Source: CAD feature listing. Evaluate the final solid. Frame: model axes, mm. Give positions to 0.01 mm unless a question says otherwise; leave off trailing zeros. Answer as a JSON object with one key per item and string values. Group by question number.
1. Pin query (flat end, axial travel): P1, Ø5, axis at x = -78.5, z = -41.5, coming from the -Y side. Return the tip coordinate at first contact, or that it passes through.
2. Pull-direction query (Z, two-part tool) for faces 1 (the cylindrical face through (53.393, 71.479, 44.233)), 2 (the flat face through (-13, 73, -1)), 3 (the cylindrical face through (56.797, 71.479, 44.359)), 4 (the cylindrical face through (56.859, 71.479, -44.297)); classes: +Z half, -Z half, draft (parallel to the pull), parting line (faces both ways), or undercut.
3. Material intervals for L1, parallel to X at y = 72.05, z = 41.5; L2, parallel to Z at x = -78.5, y = 72.05, sorted ascending. Write a range as [from, to].
from build123d import *

# Parameters (mm, degrees)
SKETCH1_W                 = 134.5
SKETCH1_H                 = 85
BOSS_EXTRUDE1_DEPTH       = 3
SKETCH2_W                 = 140.5
SKETCH2_H                 = 91
SKETCH2_W_2               = 134.5
SKETCH2_H_2               = 85
BOSS_EXTRUDE2_DEPTH       = 70
BOSS_EXTRUDE3_START       = 5
SKETCH3_W                 = 100
SKETCH3_H                 = 80
BOSS_EXTRUDE3_DEPTH       = 5
SKETCH5_W                 = 3
SKETCH5_H                 = 66
BOSS_EXTRUDE5_DEPTH       = 30
SKETCH6_R                 = 3
SKETCH6_R_2               = 1
BOSS_EXTRUDE6_DEPTH       = 10
SKETCH7_W                 = 100
SKETCH7_H                 = 80
CUT_EXTRUDE2_DEPTH        = 10
SKETCH6_2_R               = 3
SKETCH6_2_R_2             = 1
BOSS_EXTRUDE7_DEPTH       = 8
MIRROR4_COPY_1_SKETCH_R   = 3
MIRROR4_COPY_1_SKETCH_R_2 = 1
MIRROR4_COPY_1_DEPTH      = 8
SKETCH9_R                 = 26.15
SKETCH9_W                 = 29.3
SKETCH9_H                 = 26.2
SKETCH9_R_2               = 1
SKETCH9_R_3               = 3.4
SKETCH9_R_4               = 7.9
CUT_EXTRUDE3_DEPTH        = 3
SKETCH10_R                = 2.95
SKETCH10_R_2              = 5.9
CUT_EXTRUDE4_DEPTH        = 3
BOSS_EXTRUDE8_DEPTH       = 7
FILLET1_R                 = 4
CUT_EXTRUDE6_DEPTH        = 5
SKETCH14_R                = 2.8
BOSS_EXTRUDE9_DEPTH       = 3


with BuildPart() as part:
    # Sketch1 → Boss-Extrude1 (new body)
    with BuildSketch(Plane(origin=(0, 0, 0), x_dir=(1, 0, 0), z_dir=(0, 1, 0))):
        with Locations((-12.25, 0)):
            Rectangle(SKETCH1_W, SKETCH1_H)
    extrude(amount=BOSS_EXTRUDE1_DEPTH)

    # Sketch2 → Boss-Extrude2 (add)
    with BuildSketch(Plane(origin=(0, 0, 0), x_dir=(1, 0, 0), z_dir=(0, 1, 0))):
        with Locations((-12.25, 0)):
            Rectangle(SKETCH2_W, SKETCH2_H)
        with Locations((-12.25, 0)):
            Rectangle(SKETCH2_W_2, SKETCH2_H_2, mode=Mode.SUBTRACT)
    extrude(amount=BOSS_EXTRUDE2_DEPTH)

    # Sketch5 → Boss-Extrude5 (add)
    with BuildSketch(Plane(origin=(0, 3, 0), x_dir=(1, 0, 0), z_dir=(0, 1, 0))):
        Polygon((-58, -26.5), (-58, -23.5), (-61, -23.5), (-79.5, -23.5), (-79.5, -26.5), align=None)
        with Locations((-59.5, 9.5)):
            Rectangle(SKETCH5_W, SKETCH5_H)
    extrude(amount=BOSS_EXTRUDE5_DEPTH)



with BuildPart() as body_2:
    # Sketch3 → Boss-Extrude3 (new body)
    with BuildSketch(Plane(origin=(0, 3, 0), x_dir=(1, 0, 0), z_dir=(0, 1, 0)).offset(BOSS_EXTRUDE3_START)):
        Rectangle(SKETCH3_W, SKETCH3_H)
    extrude(amount=BOSS_EXTRUDE3_DEPTH)


with BuildPart() as part_1:
    add(part.part)

    add(body_2.part)  # Boss-Extrude6 merges body 2
    # Sketch6 → Boss-Extrude6 (add)
    with BuildSketch(Plane(origin=(0, 3, 0), x_dir=(1, 0, 0), z_dir=(0, 1, 0))):
        with Locations((-45, -35)):
            Circle(SKETCH6_R)
        with Locations((-45, -35)):
            Circle(SKETCH6_R_2, mode=Mode.SUBTRACT)
    extrude(amount=BOSS_EXTRUDE6_DEPTH)

    # Sketch7 → Cut-Extrude2 (cut)
    with BuildSketch(Plane(origin=(0, 13, 0), x_dir=(1, 0, 0), z_dir=(0, 1, 0))):
        Rectangle(SKETCH7_W, SKETCH7_H)
    extrude(amount=-CUT_EXTRUDE2_DEPTH, mode=Mode.SUBTRACT)

    # Sketch6<2> → Boss-Extrude7 (add)
    with BuildSketch(Plane(origin=(0, 3, 0), x_dir=(1, 0, 0), z_dir=(0, 1, 0))):
        with Locations((-45, -35)):
            Circle(SKETCH6_2_R)
        with Locations((-45, -35)):
            Circle(SKETCH6_2_R_2, mode=Mode.SUBTRACT)
    boss_extrude7 = extrude(amount=BOSS_EXTRUDE7_DEPTH)

    # Mirror3: Boss-Extrude7 across plane
    add(boss_extrude7.mirror(Plane.XY))

    # Mirror4: Boss-Extrude7 across plane
    add(boss_extrude7.mirror(Plane(origin=(0, 0, 0), x_dir=(0, 0, 1), z_dir=(1, 0, 0))))

    # Mirror4 copy 1 sketch → Mirror4 copy 1 (add)
    with BuildSketch(Plane(origin=(0, 3, 0), x_dir=(-1, 0, 0), z_dir=(0, 1, 0))):
        with Locations((-45, -35)):
            Circle(MIRROR4_COPY_1_SKETCH_R)
        with Locations((-45, -35)):
            Circle(MIRROR4_COPY_1_SKETCH_R_2, mode=Mode.SUBTRACT)
    extrude(amount=MIRROR4_COPY_1_DEPTH)

    # Sketch9 → Cut-Extrude3 (cut)
    with BuildSketch(Plane.XY.offset(45.5)):
        with Locations((23, 40.85)):
            Circle(SKETCH9_R)
        with Locations((-47.5, 50)):
            Rectangle(SKETCH9_W, SKETCH9_H)
        with Locations((1.786796564, 62.063203436)):
            Circle(SKETCH9_R_2)
        with Locations((44.213203436, 62.063203436)):
            Circle(SKETCH9_R_2)
        with Locations((44.213203436, 19.636796564)):
            Circle(SKETCH9_R_2)
        with Locations((1.786796564, 19.636796564)):
            Circle(SKETCH9_R_2)
        with Locations((-58.75, 21.9)):
            Circle(SKETCH9_R_3)
        with Locations((-40.75, 21.9)):
            Circle(SKETCH9_R_4)
    extrude(amount=-CUT_EXTRUDE3_DEPTH, mode=Mode.SUBTRACT)

    # Sketch10 → Cut-Extrude4 (cut)
    with BuildSketch(Plane(origin=(58, 0, 0), x_dir=(0, 0, -1), z_dir=(1, 0, 0))):
        with Locations((15.5, 55)):
            Circle(SKETCH10_R)
        with Locations((30.5, 55)):
            Circle(SKETCH10_R_2)
    extrude(amount=-CUT_EXTRUDE4_DEPTH, mode=Mode.SUBTRACT)

    # Sketch11 → Boss-Extrude8 (add)
    with BuildSketch(Plane(origin=(0, 70, 0), x_dir=(1, 0, 0), z_dir=(0, 1, 0))):
        Polygon((-74.5, 42.5), (-79.5, 42.5), (-79.5, 37.5), align=None)
        Polygon((55, 37.5), (55, 42.5), (50, 42.5), align=None)
        Polygon((50, -42.5), (55, -42.5), (55, -37.5), align=None)
        Polygon((-79.5, -37.5), (-79.5, -42.5), (-74.5, -42.5), align=None)
    extrude(amount=-BOSS_EXTRUDE8_DEPTH)

    # Fillet1
    fillet1_edges = [part_1.edges().sort_by_distance(p)[0] for p in [
        (58, 35, 45.5),
        (58, 35, -45.5),
        (-82.5, 35, -45.5),
        (-82.5, 35, 45.5),
    ]]
    fillet(fillet1_edges, radius=FILLET1_R)

    # Sketch13 → Cut-Extrude6 (cut)
    with BuildSketch(Plane(origin=(0, 70, 0), x_dir=(1, 0, 0), z_dir=(0, 1, 0))):
        with BuildLine():
            ThreePointArc((55.371320344, 42.871320344), (53.957106781, 42.871320344), (53.957106781, 41.457106781))
            Line((53.957106781, 41.457106781), (55.371320344, 42.871320344))
        make_face()
        with BuildLine():
            Line((55.371320344, 42.871320344), (53.957106781, 41.457106781))
            ThreePointArc((53.957106781, 41.457106781), (55.046896995, 41.24033403), (55.664213562, 42.164213562))
            ThreePointArc((55.664213562, 42.164213562), (55.588093095, 42.546896995), (55.371320344, 42.871320344))
        make_face()
        with BuildLine():
            ThreePointArc((53.957106781, -41.457106781), (53.957106781, -42.871320344), (55.371320344, -42.871320344))
            Line((55.371320344, -42.871320344), (53.957106781, -41.457106781))
        make_face()
        with BuildLine():
            Line((53.957106781, -41.457106781), (55.371320344, -42.871320344))
            ThreePointArc((55.371320344, -42.871320344), (55.588093095, -42.546896995), (55.664213562, -42.164213562))
            ThreePointArc((55.664213562, -42.164213562), (55.046896995, -41.24033403), (53.957106781, -41.457106781))
        make_face()
        with BuildLine():
            ThreePointArc((-78.164213562, -42.164213562), (-78.24033403, -41.78153013), (-78.457106781, -41.457106781))
            Line((-78.457106781, -41.457106781), (-79.871320344, -42.871320344))
            ThreePointArc((-79.871320344, -42.871320344), (-78.78153013, -43.088093095), (-78.164213562, -42.164213562))
        make_face()
        with BuildLine():
            Line((-79.871320344, -42.871320344), (-78.457106781, -41.457106781))
            ThreePointArc((-78.457106781, -41.457106781), (-79.871320344, -41.457106781), (-79.871320344, -42.871320344))
        make_face()
        with BuildLine():
            ThreePointArc((-78.164213562, 42.164213562), (-78.78153013, 43.088093095), (-79.871320344, 42.871320344))
            Line((-79.871320344, 42.871320344), (-78.457106781, 41.457106781))
            ThreePointArc((-78.457106781, 41.457106781), (-78.24033403, 41.78153013), (-78.164213562, 42.164213562))
        make_face()
        with BuildLine():
            Line((-78.457106781, 41.457106781), (-79.871320344, 42.871320344))
            ThreePointArc((-79.871320344, 42.871320344), (-79.871320344, 41.457106781), (-78.457106781, 41.457106781))
        make_face()
    extrude(amount=-CUT_EXTRUDE6_DEPTH, mode=Mode.SUBTRACT)


with BuildPart() as body_2_2:
    # Sketch14 → Boss-Extrude9 (new body)
    with BuildSketch(Plane(origin=(0, 70, 0), x_dir=(1, 0, 0), z_dir=(0, 1, 0))):
        with BuildLine():
            Line((-78.5, -45.5), (54, -45.5))
            ThreePointArc((54, -45.5), (56.828427125, -44.328427125), (58, -41.5))
            Line((58, -41.5), (58, 41.5))
            ThreePointArc((58, 41.5), (56.828427125, 44.328427125), (54, 45.5))
            Line((54, 45.5), (-78.5, 45.5))
            ThreePointArc((-78.5, 45.5), (-81.328427125, 44.328427125), (-82.5, 41.5))
            Line((-82.5, 41.5), (-82.5, -41.5))
            ThreePointArc((-82.5, -41.5), (-81.328427125, -44.328427125), (-78.5, -45.5))
        make_face()
        with Locations((-78.5, 41.5)):
            Circle(SKETCH14_R, mode=Mode.SUBTRACT)
        with Locations((54, 41.5)):
            Circle(SKETCH14_R, mode=Mode.SUBTRACT)
        with Locations((54, -41.5)):
            Circle(SKETCH14_R, mode=Mode.SUBTRACT)
        with Locations((-78.5, -41.5)):
            Circle(SKETCH14_R, mode=Mode.SUBTRACT)
    extrude(amount=BOSS_EXTRUDE9_DEPTH)


solid = body_2_2.part
Answer sheet:
{
 "1": {"P1": "through"},
 "2": {"face 1": "undercut", "face 2": "draft", "face 3": "+Z half", "face 4": "-Z half"},
 "3": {"L1": "[-82.5, -81.3], [-75.7, 51.2], [56.8, 58]", "L2": "[-45.5, -44.3], [-38.7, 38.7], [44.3, 45.5]"}
}
